```python
from build123d import *

# Parameters (mm, degrees)
SKETCH1_W           = 22
SKETCH1_H           = 53
BOSS_EXTRUDE1_DEPTH = 3
SKETCH2_W           = 22
SKETCH2_H           = 3
BOSS_EXTRUDE2_DEPTH = 22
SKETCH3_R           = 1.75
CUT_EXTRUDE1_DEPTH  = 22
SKETCH4_R           = 1.75
CUT_EXTRUDE2_DEPTH  = 63.593929418
SKETCH5_W           = 20
SKETCH5_H           = 30
BOSS_EXTRUDE3_DEPTH = 5
BOSS_EXTRUDE4_DEPTH = 30
SKETCH7_R           = 4
CUT_EXTRUDE3_DEPTH  = 20
BOSS_EXTRUDE5_START = 1
SKETCH8_W           = 22
SKETCH8_H           = 23
SKETCH8_R           = 1.75
BOSS_EXTRUDE5_DEPTH = 1
BOSS_EXTRUDE6_START = 1
SKETCH9_W           = 22
SKETCH9_H           = 26
SKETCH9_R           = 1.75
BOSS_EXTRUDE6_DEPTH = 1
BOSS_EXTRUDE7_START = 1
SKETCH10_W          = 22
SKETCH10_H          = 26
SKETCH10_R          = 1.75
BOSS_EXTRUDE7_DEPTH = 1
BOSS_EXTRUDE8_START = 1
SKETCH11_W          = 22
SKETCH11_H          = 25
SKETCH11_R          = 1.75
BOSS_EXTRUDE8_DEPTH = 1
FILLET1_R           = 2
FILLET2_R           = 2


with BuildPart() as part:
    # Sketch1 → Boss-Extrude1 (new body)
    with BuildSketch(Plane.XY):
        with Locations((11, 26.5)):
            Rectangle(SKETCH1_W, SKETCH1_H)
    extrude(amount=BOSS_EXTRUDE1_DEPTH)

    # Sketch2 → Boss-Extrude2 (add)
    with BuildSketch(Plane.XY.offset(3)):
        with Locations((11, 1.5)):
            Rectangle(SKETCH2_W, SKETCH2_H)
    extrude(amount=BOSS_EXTRUDE2_DEPTH)

    # Sketch3 → Cut-Extrude1 (cut)
    with BuildSketch(Plane.XZ):
        with Locations(Location((7.5, 15, 0), (0, 0, 270))):
            Circle(SKETCH3_R)
    extrude(amount=-CUT_EXTRUDE1_DEPTH, mode=Mode.SUBTRACT)

    # Sketch4 → Cut-Extrude2 (cut, through all)
    with BuildSketch(Plane(origin=(0, 0, 0), x_dir=(-1, 0, 0), z_dir=(0, 0, -1))):
        with Locations((-7.5, 15)):
            Circle(SKETCH4_R)
    extrude(amount=-CUT_EXTRUDE2_DEPTH, mode=Mode.SUBTRACT)

    # Sketch5 → Boss-Extrude3 (add)
    with BuildSketch(Plane(origin=(0, 0, 0), x_dir=(-1, 0, 0), z_dir=(0, 0, -1))):
        with Locations((-12, 38)):
            Rectangle(SKETCH5_W, SKETCH5_H)
    extrude(amount=BOSS_EXTRUDE3_DEPTH)

    # Sketch6 → Boss-Extrude4 (add)
    with BuildSketch(Plane.XZ.offset(-23)):
        with BuildLine():
            Line((19.5, -5), (4.5, -5))
            ThreePointArc((4.5, -5), (12, -12.5), (19.5, -5))
        make_face()
    extrude(amount=-BOSS_EXTRUDE4_DEPTH)

    # Sketch7 → Cut-Extrude3 (cut)
    with BuildSketch(Plane(origin=(0, 53, 0), x_dir=(1, 0, 0), z_dir=(0, 1, 0))):
        with Locations(Location((12, 5, 0), (0, 0, 270))):
            Circle(SKETCH7_R)
    extrude(amount=-CUT_EXTRUDE3_DEPTH, mode=Mode.SUBTRACT)

    # Sketch8 → Boss-Extrude5 (add)
    with BuildSketch(Plane(origin=(0, 0, 0), x_dir=(-1, 0, 0), z_dir=(0, 0, -1)).offset(BOSS_EXTRUDE5_START)):
        with Locations((-11, 11.5)):
            Rectangle(SKETCH8_W, SKETCH8_H)
        with Locations((-7.5, 15)):
            Circle(SKETCH8_R, mode=Mode.SUBTRACT)
    extrude(amount=-BOSS_EXTRUDE5_DEPTH)

    # Sketch9 → Boss-Extrude6 (add)
    with BuildSketch(Plane.XZ.offset(BOSS_EXTRUDE6_START)):
        with Locations((11, 12)):
            Rectangle(SKETCH9_W, SKETCH9_H)
        with Locations(Location((7.5, 15, 0), (0, 0, 270))):
            Circle(SKETCH9_R, mode=Mode.SUBTRACT)
    extrude(amount=-BOSS_EXTRUDE6_DEPTH)

    # Sketch10 → Boss-Extrude7 (add)
    with BuildSketch(Plane(origin=(0, -1, 0), x_dir=(-1, 0, 0), z_dir=(0, -1, 0)).offset(BOSS_EXTRUDE7_START)):
        with Locations((-11, -12)):
            Rectangle(SKETCH10_W, SKETCH10_H)
        with Locations(Location((-7.5, -15, 0), (0, 0, 90))):
            Circle(SKETCH10_R, mode=Mode.SUBTRACT)
    extrude(amount=-BOSS_EXTRUDE7_DEPTH)

    # Sketch11 → Boss-Extrude8 (add)
    with BuildSketch(Plane(origin=(0, 0, -1), x_dir=(-1, 0, 0), z_dir=(0, 0, -1)).offset(BOSS_EXTRUDE8_START)):
        with Locations((-11, 10.5)):
            Rectangle(SKETCH11_W, SKETCH11_H)
        with Locations((-7.5, 15)):
            Circle(SKETCH11_R, mode=Mode.SUBTRACT)
    extrude(amount=-BOSS_EXTRUDE8_DEPTH)

    # Fillet1
    fillet1_edges = [part.edges().sort_by_distance(p)[0] for p in [
        (11, -2, -2),
    ]]
    fillet(fillet1_edges, radius=FILLET1_R)

    # Fillet2
    fillet2_edges = [part.edges().sort_by_distance(p)[0] for p in [
        (12, 23, -2),
    ]]
    fillet(fillet2_edges, radius=FILLET2_R)


solid = part.part
```
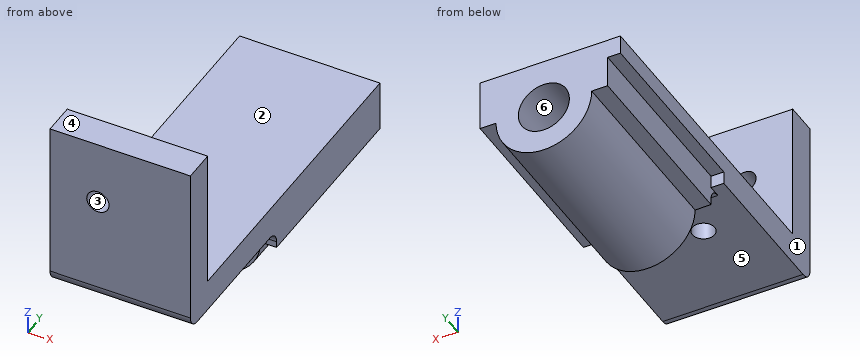
Source: CAD feature listing. Evaluate the final solid. Frame: model axes, mm. Face numbers are marked on the shaded views. A direction names the side the tool comes from. Round coordinates to 2 decimals unless told otherwise and drop trailing zeros. Loops run counter-clockwise (first coordinate to the right, second up) from the corner with the lowest first, then second, coordinate; pieces in that order, holes last. Notation, with made-up numbers: M 40.5,71.5 L 64.5,71.5 A9 cw 64.5,80.5 Z; hole C -19,50.25 d2. An arc over 180 degrees is marked long. Use a Markdown table: item, result. Add a question column.
1. Section query C-C on z = 14.5. Return the cut outline in (x, y).
2. Contact query for flat-ended pins moving along their axis: P1, Ø4, axis at x = 13, z = -5, coming from the +Y side; P2, Ø4, axis at x = 16.5, y = 12, coming from the +Z side; P3, Ø4, axis at x = 9, z = -8.5, coming from the -Y side; P4, Ø3, axis at x = 7.5, y = 15, coming from the -Z side. Output: stop coordinate, or through.
3. Section query D-D on y = 44.5. Return the cut outline in (x, z).
4. Section query A-A on y = 15. Return the cut outline in (x, z).
5. Section query B-B on x = 3.75. Return the cut outline in (y, z), then the cut area to 3 significant figures.
6. Mould query, pull axis Z, two halves, no side actions, for the marked faces 3, 4, 5 and 6. Classes: pulls with the +Z half, pulls with the -Z half, needs draft (parallel to the pull), parting line crosses it, or undercut.
7. Reachability of the marked faces 1 and 2 from +Z, -Z, +X, -X, +Y, -Y: full face, straight path, thin tool, end or side. Return the list, or none.
8. Line query: line 1 (Y direction, x = 7.5, z = 0.95); line 2 (X direction, y = 1.1, z = 15); line 3 (Y direction, x = 1.25, z = 4). Output: solid intervals per line, ascending.
Reported:
| question | item | result |
|---|---|---|
| 1 | outline | M 0,-2 L 5.82,-2 L 5.82,3 L 0,3 Z; M 9.18,-2 L 22,-2 L 22,3 L 9.18,3 Z |
| 2 | P1 | stops at y = 33 |
| 2 | P2 | stops at z = 3 |
| 2 | P3 | stops at y = 23 |
| 2 | P4 | passes through |
| 3 | outline | M 0,0 L 2,0 L 2,-5 L 4.5,-5 A7.5 ccw 19.5,-5 L 22,-5 L 22,3 L 0,3 Z; hole C 12,-5 d8 |
| 4 | outline | M 0,-2 L 5.75,-2 L 5.75,3 L 0,3 Z; M 9.25,-2 L 22,-2 L 22,3 L 9.25,3 Z |
| 5 | outline | M -2,0 A2 ccw 0,-2 L 21,-2 A2 cw 23,-4 L 23,-5 L 53,-5 L 53,3 L 3,3 L 3,25 L -2,25 Z |
| 5 | area | 475 mm² |
| 6 | face 3 | undercut |
| 6 | face 4 | pulls with the +Z half |
| 6 | face 5 | pulls with the -Z half |
| 6 | face 6 | undercut |
| 7 | face 1 | +Z, -Z, -X, +Y, -Y |
| 7 | face 2 | +Z, +X, -X, +Y |
| 8 | line 1 | y = -2 to 13.25, 16.75 to 53 |
| 8 | line 2 | x = 0 to 5.75, 9.25 to 22 |
| 8 | line 3 | y = -2 to 3 |
